from build123d import *

# Parameters (mm, degrees)
BOSS_EXTRUDE1_DEPTH      = 1
BOSS_EXTRUDE1_DEPTH_BACK = 1.5
SKETCH1_R                = 3.5
SKETCH1_R_2              = 1.625
SKETCH2_R                = 5.5
BOSS_EXTRUDE2_DEPTH      = 3.2
SKETCH3_R                = 4.1
CUT_EXTRUDE1_DEPTH       = 2.9
SKETCH4_R                = 1.65
CUT_EXTRUDE2_DEPTH       = 10
FILLET2_R                = 2
SKETCH5_R                = 4.5
CUT_EXTRUDE3_DEPTH       = 0.5


with BuildPart() as part:
    # Sketch1 → Boss-Extrude1 (new, two sides: drawn at the far end of the back side and taken through both)
    with BuildSketch(Plane.XY.offset(-BOSS_EXTRUDE1_DEPTH_BACK)):
        Circle(SKETCH1_R)
        Circle(SKETCH1_R_2, mode=Mode.SUBTRACT)
    extrude(amount=BOSS_EXTRUDE1_DEPTH + BOSS_EXTRUDE1_DEPTH_BACK)

    # Sketch2 → Boss-Extrude2 (add)
    with BuildSketch(Plane.XY.offset(1)):
        Circle(SKETCH2_R)
    extrude(amount=BOSS_EXTRUDE2_DEPTH)

    # Sketch3 → Cut-Extrude1 (cut)
    with BuildSketch(Plane.XY.offset(4.2)):
        Circle(SKETCH3_R)
    extrude(amount=-CUT_EXTRUDE1_DEPTH, mode=Mode.SUBTRACT)

    # Sketch4 → Cut-Extrude2 (cut)
    with BuildSketch(Plane(origin=(0, 0, -1.5), x_dir=(-1, 0, 0), z_dir=(0, 0, -1))):
        Circle(SKETCH4_R)
    extrude(amount=-CUT_EXTRUDE2_DEPTH, mode=Mode.SUBTRACT)

    # Fillet2
    # the kernel refuses this fillet: 2 mm, written as the material it adds along each edge
    with BuildSketch(Plane(origin=(0, 0, 1), x_dir=(1, 0, 0), z_dir=(0, -1, 0))) as fillet2_piece_1:
        with BuildLine():
            CenterArc((3.5 + FILLET2_R, -FILLET2_R), FILLET2_R, 90, 90)
            Line((3.5, -FILLET2_R), (3.5, 0))
            Line((3.5, 0), (3.5 + FILLET2_R, 0))
        make_face()
    revolve(axis=Axis((0, 0, 1), (0, 0, 1)))

    # Sketch5 → Cut-Extrude3 (cut)
    with BuildSketch(Plane.XY.offset(1.3)):
        Circle(SKETCH5_R)
    extrude(amount=CUT_EXTRUDE3_DEPTH, mode=Mode.SUBTRACT)


solid = part.part
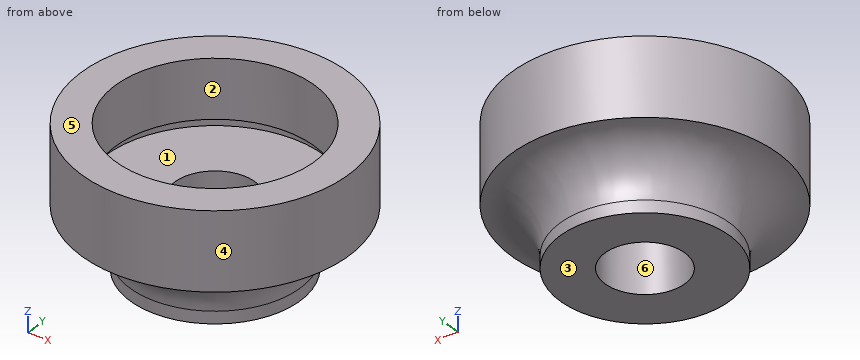
Can you work these out from the model? Positions are in its coordinate system, mm. Face numbers are marked on the shaded views. A direction names the side the tool comes from. Coordinates: 2 decimals unless noted, no trailing zeros. Loops run counter-clockwise (first coordinate to the right, second up) from the corner with the lowest first, then second, coordinate; pieces in that order, holes last. Notation, with made-up numbers: (60.5, -33) - (83.5, -33) arc R19 cw to (83.5, 3) - close; hole circle Ø6 at (78, 42). An arc over 180 degrees is marked (long way). Answer as a JSON object with one key per item and string values. Group by question number.
Item 1: For pin 1 (1.5 mm diameter, centred on y = -1.5, z = 1, fed in from +X); pin 2 (5.5 mm diameter, centred on x = 0, y = 0, fed in from +Z), each with a flat end and sliding along its axis, tell me the tip position at first contact or that it passes through.
Item 2: If we section it at A-A (x = 0): List the corners of the cut face in (y, z) for me, plus the area to 3 significant figures.
Item 3: On a 3-axis mill with a long thin cutter (end or side, diameter ignored), from which of +Z, -Z, +X, -X, +Y, -Y can I reach the whole of each face in a straight line? I mean the marked faces 1, 2 and 3. Say none if no direction works.
Item 4: If we section it at C-C (z = 2.4): List the corners of the cut face in (x, y) for me, plus the area to 3 significant figures.
Item 5: If we mould it in two halves opening along X, with no side actions, what happens to the marked faces 4, 5 and 6? For each: released by +X, released by -X, zero draft, split by the parting line, or undercut.
Item 6: If I drill on L1, parallel to Y at x = 0, z = 1.45; L2, parallel to Y at x = 0, z = 2.8; L3, parallel to Z at x = -0.5, y = 2.5, over which ranges is the centre line in solid material (lowest first)? Write a range as from..to.
Returned:
{
 "1": {"pin 1": "stops at x = 5.45", "pin 2": "stops at z = 1.3"},
 "2": {"outline": "(-5.5, 1) arc R2 cw to (-3.5, -1) - (-3.5, -1.5) - (-1.65, -1.5) - (-1.65, 1.3) - (-4.5, 1.3) - (-4.5, 1.8) - (-4.1, 1.8) - (-4.1, 4.2) - (-5.5, 4.2) - close; (1.65, -1.5) - (3.5, -1.5) - (3.5, -1) arc R2 cw to (5.5, 1) - (5.5, 4.2) - (4.1, 4.2) - (4.1, 1.8) - (4.5, 1.8) - (4.5, 1.3) - (1.65, 1.3) - close", "area": "21.0 mm²"},
 "3": {"face 1": "none", "face 2": "+Z", "face 3": "-Z, +X, -X, +Y, -Y"},
 "4": {"outline": "circle Ø11 at (0, 0); hole circle Ø8.2 at (0, 0)", "area": "42.2 mm²"},
 "5": {"face 4": "split by the parting line", "face 5": "zero draft", "face 6": "undercut"},
 "6": {"L1": "y = -5.5..-4.5, 4.5..5.5", "L2": "y = -5.5..-4.1, 4.1..5.5", "L3": "z = -1.5..1.3"}
}
